Answer from the drawing. Dimensions are ordinates in mm from the lowest x, y and z of the part. A direction names the side the tool comes from. Round coordinates to 2 decimals unless told otherwise and drop trailing zeros. Write each loop counter-clockwise with the first axis right and the second up, starting at its lowest first coordinate (ties: lowest second). Pieces come first, ordered by that corner, then holes. Notation, with made-up numbers: (64.5, 15.5) - (117.5, 15.5) arc R18 ccw to (117.5, 28.5) - close; hole circle Ø7 at (52.25, 43.25). An arc over 180 degrees is marked (long way). Answer as CSV lines item,"result". Start each with the question number.
1) Find section C-C on x = 12. Determine the outline of the cut face in (y, z) (1 decimal).
2) Find section B-B on y = 73. Determine the outline of the cut face in (x, z) (1 decimal), then the cut area to 3 significant figures.
3) Consider line 1 along Z through (x, y) = (76, 62) (1 decimal); line 2 along Y through (x, z) = (123, 68.5) (1 decimal). Determine where each line is inside the solid, lowest interval first.
4) For a pull along Y with two mould halves and no side action, classify the marked faces 1, 2, 3 and 4 as +Y half, -Y half, draft (parallel to the pull), parting line (faces both ways), or undercut.
5) Find section A-A on z = 18.5. Determine the outline of the cut face in (x, y) (1 decimal), then the cut area to 3 significant figures.
6) Which of the six approach directions +Z, -Z, +X, -X, +Y, -Y give full straight-line access (tool end or side, diameter ignored) to the marked faces 5 and 6?
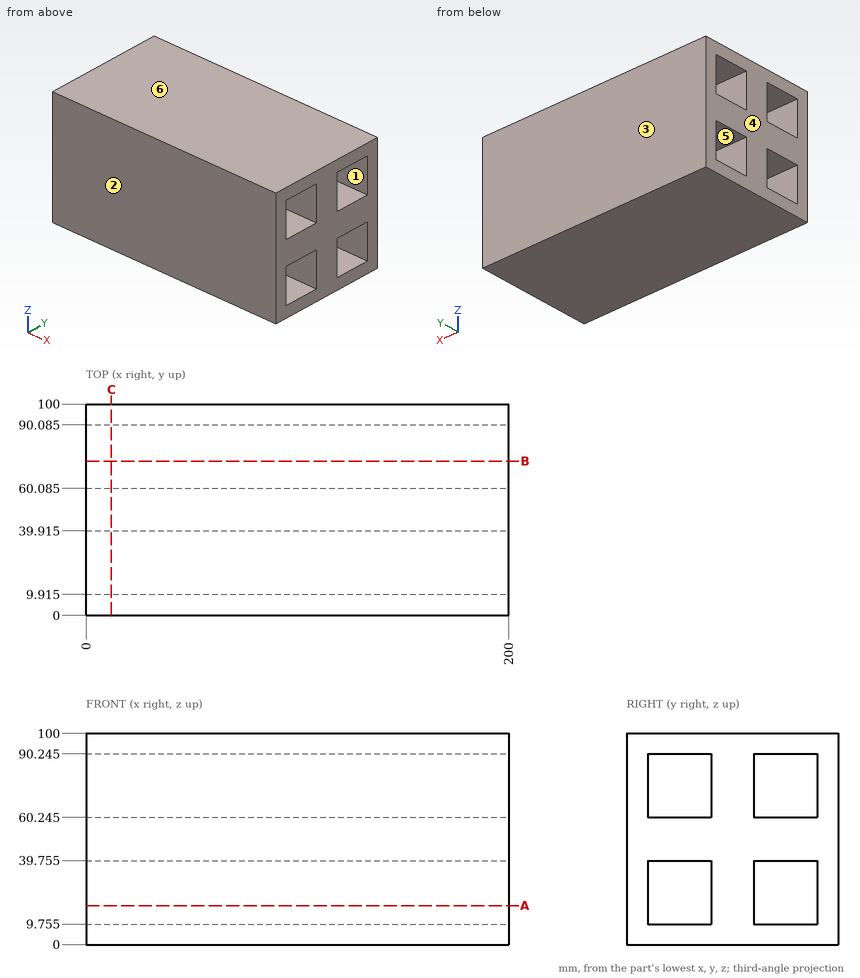
Check values:
1,outline,"(0, 0) - (100, 0) - (100, 100) - (0, 100) - close; hole (9.9, 9.8) - (39.9, 9.8) - (39.9, 39.8) - (9.9, 39.8) - close; hole (9.9, 60.2) - (39.9, 60.2) - (39.9, 90.2) - (9.9, 90.2) - close; hole (60.1, 9.8) - (90.1, 9.8) - (90.1, 39.8) - (60.1, 39.8) - close; hole (60.1, 60.2) - (90.1, 60.2) - (90.1, 90.2) - (60.1, 90.2) - close"
2,outline,"(0, 0) - (200, 0) - (200, 9.8) - (0, 9.8) - close; (0, 39.8) - (200, 39.8) - (200, 60.2) - (0, 60.2) - close; (0, 90.2) - (200, 90.2) - (200, 100) - (0, 100) - close"
2,area,"8,000 mm^2"
3,line 1,"z = 0 to 9.8, 39.8 to 60.2, 90.2 to 100"
3,line 2,"y = 0 to 9.9, 39.9 to 60.1, 90.1 to 100"
4,face 1,"undercut"
4,face 2,"-Y half"
4,face 3,"+Y half"
4,face 4,"draft"
5,outline,"(0, 0) - (200, 0) - (200, 9.9) - (0, 9.9) - close; (0, 39.9) - (200, 39.9) - (200, 60.1) - (0, 60.1) - close; (0, 90.1) - (200, 90.1) - (200, 100) - (0, 100) - close"
5,area,"8,000 mm^2"
6,face 5,"+X, -X"
6,face 6,"+Z, +X, -X, +Y, -Y"
